Work out the finished part from the listing and answer in its coordinate system (mm). Face numbers are marked on the shaded views. A direction names the side the tool comes from. Give positions to 0.01 mm unless a question says otherwise; leave off trailing zeros. Order: outer loops, then holes, each group sorted by start corner. A loop starts at its lowest first (then second) coordinate and runs counter-clockwise, first axis right, second up. Notation, with made-up numbers: (-37.5, 47.25) -> (8.5, 47.25) arc R27 ccw to (8.5, 85.25) -> close; hole circle Ø10 at (-25.75, 46.5). An arc over 180 degrees is marked (long way). Answer as CSV lines item,"result". Start each with the question number.
1. Flat-ended cylindrical pins translate along their axes: pin 1 (12 mm diameter, centred on y = 34, z = 12.5, fed in from -X); pin 2 (1 mm diameter, centred on x = 53.5, z = 13, fed in from -Y); pin 3 (0.6 mm diameter, centred on x = -1, z = 32, fed in from +Y). Find the tip coordinate at first contact, or state that the pin passes through.
2. For the marked faces 1 and 2, determine the directions among +Z, -Z, +X, -X, +Y, -Y from which every point of the face is accessible in a straight line to the end or side of a thin tool.
3. A cutting plane is placed at A-A (y = 81). Give the vertices of the cut face in (x, z).
4. Find the intervals of material crossed by L1, parallel to Z at x = 7.5, y = 23; L2, parallel to Y at x = 84, z = 27, in increasing order.
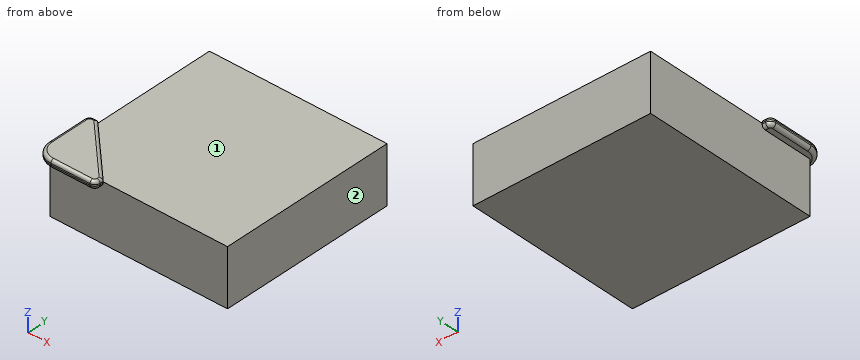
from build123d import *

# Parameters (mm, degrees)
F0_W     = 100
F0_H     = 100
F1_DEPTH = 32
F3_DEPTH = 2
F4_DEPTH = 2.5
F5_R     = 2
F6_R     = 1.689949


with BuildPart() as f1:
    # F0 (on Top) → F1 (new body)
    with BuildSketch(Plane.XY):
        with Locations((50, 50)):
            Rectangle(F0_W, F0_H)
    extrude(amount=F1_DEPTH)



with BuildPart() as f3:
    # F2 (on face) → F3 (new body)
    with BuildSketch(Plane.XY.offset(32)):
        Polygon((0, 30), (0, 0), (30, 0), align=None)
        with BuildLine():
            Line((30, 0), (0, 0))
            Line((0, 0), (0, 30))
            Line((0, 30), (-2, 30))
            ThreePointArc((-2, 30), (-4.12132, 29.12132), (-5, 27))
            Line((-5, 27), (-5, 5))
            ThreePointArc((-5, 5), (-2.071068, -2.071068), (5, -5))
            Line((5, -5), (27.016253, -5))
            ThreePointArc((27.016253, -5), (29.146228, -4.11263), (30.016152, -1.975471))
            Line((30.016152, -1.975471), (30, 0))
        make_face()
    extrude(amount=F3_DEPTH)


with BuildPart() as f1_1:
    add(f1.part)

    add(f3.part)  # F4 merges F3
    # F2 (on face) → F4 (join)
    with BuildSketch(Plane.XY.offset(32)):
        with BuildLine():
            Line((30, 0), (0, 0))
            Line((0, 0), (0, 30))
            Line((0, 30), (-2, 30))
            ThreePointArc((-2, 30), (-4.12132, 29.12132), (-5, 27))
            Line((-5, 27), (-5, 5))
            ThreePointArc((-5, 5), (-2.071068, -2.071068), (5, -5))
            Line((5, -5), (27.016253, -5))
            ThreePointArc((27.016253, -5), (29.146228, -4.11263), (30.016152, -1.975471))
            Line((30.016152, -1.975471), (30, 0))
        make_face()
    extrude(amount=-F4_DEPTH)

    # F5
    f5_edges = [f1_1.edges().sort_by_distance(p)[0] for p in [
        (-1, 30, 29.5),
        (-4.12132, 29.12132, 29.5),
        (-5, 16, 29.5),
        (-2.071068, -2.071068, 29.5),
        (16.008126, -5, 29.5),
        (29.146228, -4.11263, 29.5),
        (30.008076, -0.987736, 29.5),
    ]]
    fillet(f5_edges, radius=F5_R)

    # F6
    f6_edges = [f1_1.edges().sort_by_distance(p)[0] for p in [
        (15, 15, 34),
        (-1, 30, 34),
        (-4.12132, 29.12132, 34),
        (-5, 16, 34),
        (-2.071068, -2.071068, 34),
        (16.008126, -5, 34),
        (29.146228, -4.11263, 34),
        (30.008076, -0.987736, 34),
    ]]
    fillet(f6_edges, radius=F6_R)


solid = f1_1.part
Answer sheet:
1,pin 1,"stops at x = 0"
1,pin 2,"stops at y = 0"
1,pin 3,"stops at y = 30"
2,face 1,"+Z, +X, +Y"
2,face 2,"+Z, -Z, +X, +Y, -Y"
3,outline,"(0, 0) -> (100, 0) -> (100, 32) -> (0, 32) -> close"
4,L1,"z = 0 to 32"
4,L2,"y = 0 to 100"
